from build123d import *

# Parameters (mm, degrees)
SKETCH_R     = 1.25
SKETCH_R_2   = 12
PAD_DEPTH    = 3
SKETCH001_W  = 42.3
SKETCH001_H  = 3
PAD001_DEPTH = 48
SKETCH002_R  = 2
SKETCH002_W  = 15
SKETCH002_H  = 15
POCKET_DEPTH = 48.301


with BuildPart() as part:
    # Sketch → Pad (new body)
    with BuildSketch(Plane.XY):
        Polygon((0, 0), (42.3, 0), (42.3, 42.3), (42.3, 48.3), (0, 48.3), (0, 42.3), align=None)
        with Locations((5.65, 36.65)):
            Circle(SKETCH_R, mode=Mode.SUBTRACT)
        with Locations((36.65, 36.65)):
            Circle(SKETCH_R, mode=Mode.SUBTRACT)
        with Locations((5.65, 5.65)):
            Circle(SKETCH_R, mode=Mode.SUBTRACT)
        with Locations((36.65, 5.65)):
            Circle(SKETCH_R, mode=Mode.SUBTRACT)
        with Locations((21.15, 21.15)):
            Circle(SKETCH_R_2, mode=Mode.SUBTRACT)
    extrude(amount=PAD_DEPTH)

    # Sketch001 → Pad001 (new body)
    with BuildSketch(Plane(origin=(0, 0, 0), x_dir=(1, 0, 0), z_dir=(0, 0, -1))):
        with Locations((21.15, -46.8)):
            Rectangle(SKETCH001_W, SKETCH001_H)
    extrude(amount=PAD001_DEPTH)

    # Sketch002 → Pocket (cut, through all)
    with BuildSketch(Plane(origin=(0, 48.3, 0), x_dir=(-1, 0, 0), z_dir=(0, 1, 0))):
        with Locations((-36.3, -7)):
            Circle(SKETCH002_R)
        with Locations((-6, -7)):
            Circle(SKETCH002_R)
        with Locations((-36.3, -38)):
            Circle(SKETCH002_R)
        with Locations((-6, -38)):
            Circle(SKETCH002_R)
        with Locations((-21.15, -40.5)):
            Rectangle(SKETCH002_W, SKETCH002_H)
    extrude(amount=-POCKET_DEPTH, mode=Mode.SUBTRACT)


solid = part.part
Geometry check sheet. Reference: the model listing, model coordinates, mm. A direction names the side the tool comes from. Give positions to 0.01 mm unless a question says otherwise; leave off trailing zeros. Write each loop counter-clockwise with the first axis right and the second up, starting at its lowest first coordinate (ties: lowest second). Pieces come first, ordered by that corner, then holes.
1) Cross-section at C-C (x = 21.15). Record the boundary of the cut face in (y, z), plus the area to 3 significant figures.
Values follow:
outline: (0, 0) - (9.15, 0) - (9.15, 3) - (0, 3) - close; (33.15, 0) - (45.3, 0) - (45.3, -33) - (48.3, -33) - (48.3, 3) - (33.15, 3) - close
area: 172 mm2
2) Cross-section at B-B (y = 21.15). Record the boundary of the cut face in (x, z), plus the area to 3 significant figures.
Values follow:
outline: (0, 0) - (9.15, 0) - (9.15, 3) - (0, 3) - close; (33.15, 0) - (42.3, 0) - (42.3, 3) - (33.15, 3) - close
area: 54.9 mm2
3) Thickness scan on line 1 (Z direction, x = 6, y = 47.05); line 2 (Y direction, x = 36.65, z = 1.95); line 3 (Y direction, x = 29.5, z = -40). Record the ranges inside material, lowest first.
Values follow:
line 1: z = -48 to -40, -36 to -9, -5 to 3
line 2: y = 0 to 4.4, 6.9 to 35.4, 37.9 to 48.3
line 3: y = 45.3 to 48.3
4) Release check for a two-part mould opening along X. For faces 3 (the face through (5.49, 37.89, 1.48)), 4 (the face through (0, 46, -11)), 5 (the face through (16, 33, 0)), 6 (the face through (42.3, 46, -11)) record: released by +X, released by -X, zero draft, split by the parting line, or undercut.
Values follow:
face 3: undercut
face 4: released by -X
face 5: zero draft
face 6: released by +X
5) Cross-section at D-D (y = 5.65). Record the boundary of the cut face in (x, z).
Values follow:
outline: (0, 0) - (4.4, 0) - (4.4, 3) - (0, 3) - close; (6.9, 0) - (35.4, 0) - (35.4, 3) - (6.9, 3) - close; (37.9, 0) - (42.3, 0) - (42.3, 3) - (37.9, 3) - close
6) Go/stop test with flat-tipped pins: pin 1 Ø10 at (x, y) = (13, 10) entering from -Z; pin 2 Ø1.5 at (x, y) = (22.5, 47) entering from -Z; pin 3 Ø5 at (x, z) = (6, -7) entering from -Y. Record where each tip stops, or that it passes through.
Values follow:
pin 1: stops at z = 0
pin 2: stops at z = -33
pin 3: stops at y = 45.3
7) Cross-section at A-A (z = -42). Record the boundary of the cut face in (x, y), plus the area to 3 significant figures.
Values follow:
outline: (0, 45.3) - (13.65, 45.3) - (13.65, 48.3) - (0, 48.3) - close; (28.65, 45.3) - (42.3, 45.3) - (42.3, 48.3) - (28.65, 48.3) - close
area: 81.9 mm2
8) Set-up check for faces 1 (the face through (4.729, 6.495, 1.479)), 2 (the face through (13.65, 47, -41)): record each of +Z, -Z, +X, -X, +Y, -Y from which the full face is reachable in a straight line by a thin tool's end or side.
Values follow:
face 1: +Z, -Z
face 2: -Z, +Y, -Y
